```python
from build123d import *

# Parameters (mm, degrees)
BOSS_EXTRUDE1_DEPTH = 25.4
SKETCH1_3_W         = 355.6
SKETCH1_3_H         = 355.6
BOSS_EXTRUDE2_DEPTH = 12.7


with BuildPart() as part:
    # Sketch1 → Boss-Extrude1 (new body)
    with BuildSketch(Plane.XY):
        Polygon((-177.8, -177.8), (-177.8, 177.8), (-177.8, 203.2), (-203.2, 203.2), (-203.2, -203.2), (203.2, -203.2), (203.2, -177.8), (177.8, -177.8), align=None)
    extrude(amount=BOSS_EXTRUDE1_DEPTH)

    # Sketch1_3 → Boss-Extrude2 (add)
    with BuildSketch(Plane.XY):
        Polygon((-177.8, 203.2), (-177.8, 177.8), (177.8, 177.8), (177.8, -177.8), (203.2, -177.8), (203.2, 203.2), align=None)
        Rectangle(SKETCH1_3_W, SKETCH1_3_H)
        Polygon((-177.8, -177.8), (-177.8, 177.8), (-177.8, 203.2), (-203.2, 203.2), (-203.2, -203.2), (203.2, -203.2), (203.2, -177.8), (177.8, -177.8), align=None)
    extrude(amount=-BOSS_EXTRUDE2_DEPTH)


solid = part.part
```
Part model, mm, in its own coordinate system. A direction names the side the tool comes from. Round coordinates to 2 decimals unless told otherwise and drop trailing zeros. Loops run counter-clockwise (first coordinate to the right, second up) from the corner with the lowest first, then second, coordinate; pieces in that order, holes last.
1. Slice it at B-B (x = 40). Give the cut face in (y, z), and give its area (3 significant figures).
Solutions:
outline: (-203.2, -12.7) - (203.2, -12.7) - (203.2, 0) - (-177.8, 0) - (-177.8, 25.4) - (-203.2, 25.4) - close
area: 5,810 mm2
2. 3-axis set-ups, long thin cutter, end or side, ignore diameter. For faces 4 (the face through (-177.8, 10, 13)), 5 (the face through (-182, -89, 25.4)): which of +Z, -Z, +X, -X, +Y, -Y reach the whole face in a straight line?
Solutions:
face 4: +Z, +X, +Y
face 5: +Z, +X, -X, +Y, -Y
3. Two-plate mould, pull along Y, no slides. Class faces 1 (the face through (-203.2, 3, 7)), 2 (the face through (-3, -203.2, 7)), 3 (the face through (-29, 203.2, -5)): pulls with the +Y half, pulls with the -Y half, needs draft (parallel to the pull), parting line crosses it, or undercut.
Solutions:
face 1: needs draft
face 2: pulls with the -Y half
face 3: pulls with the +Y half
4. Drill centre lines: line 1 along Z through (x, y) = (-20.5, -117.5); line 2 along Y through (x, z) = (-6.5, 1.5). Where is each one in solid material? Low to high.
Solutions:
line 1: z = -12.7 to 0
line 2: y = -203.2 to -177.8
5. Flat gauge pins, fed straight in: pin 1 (12.5 mm diameter, centred on y = -26.5, z = 14.5, fed in from +X); pin 2 (20.5 mm diameter, centred on x = 34, z = 13, fed in from +Y). Where does each tip first touch, or does it go through?
Solutions:
pin 1: stops at x = -177.8
pin 2: stops at y = -177.8
6. Slice it at A-A (z = 17). Give the cut face in (x, y).
Solutions:
outline: (-203.2, -203.2) - (203.2, -203.2) - (203.2, -177.8) - (-177.8, -177.8) - (-177.8, 203.2) - (-203.2, 203.2) - close
